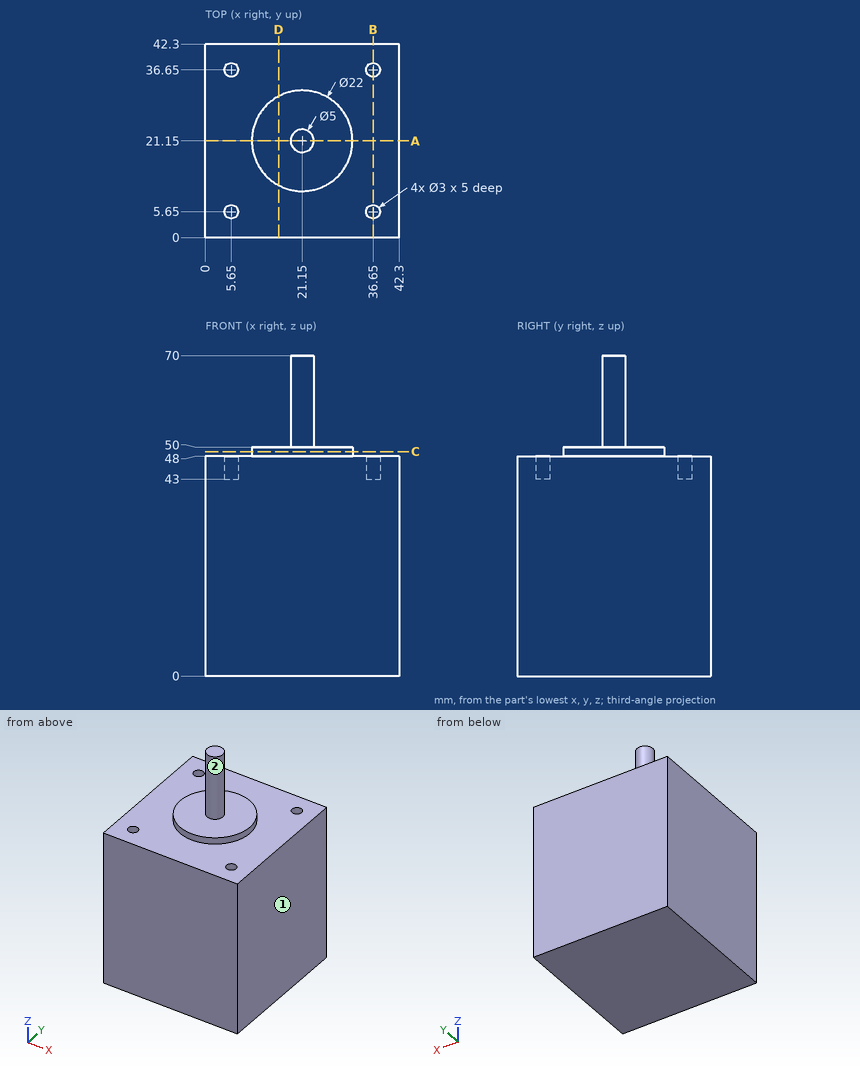
Answer from the drawing. Dimensions are ordinates in mm from the lowest x, y and z of the part. A direction names the side the tool comes from. Round coordinates to 2 decimals unless told otherwise and drop trailing zeros. Write each loop counter-clockwise with the first axis right and the second up, starting at its lowest first coordinate (ties: lowest second). Pieces come first, ordered by that corner, then holes. Notation, with made-up numbers: (27, 69) -> (46, 69) arc R23 ccw to (46, 98) -> close; hole circle Ø11 at (4.25, 88). An arc over 180 degrees is marked (long way). Answer in a Markdown table with one row per item. Add a question column.
1) Find section D-D, the plane x = 16. Determine the outline of the cut face in (y, z).
2) Find section A-A, the plane y = 21.15. Determine the outline of the cut face in (x, z), and give its area (3 significant figures).
3) Find section B-B, the plane x = 36.65. Determine the outline of the cut face in (y, z).
4) Given P1, Ø10, axis at y = 11, z = 52.5, coming from the +X side; P2, Ø8, axis at x = 22, y = 13, coming from the +Z side; P3, Ø4, axis at y = 26, z = 59.5, coming from the -X side; P4, Ø2.5, axis at x = 36.65, y = 36.65, coming from the +Z side, each flat-ended and moving along its own axis, determine where each tip first touches the part or whether it passes through.
5) Which of the six approach directions +Z, -Z, +X, -X, +Y, -Y give full straight-line access (tool end or side, diameter ignored) to the marked faces 1 and 2?
6) Consider line 1 (Y direction, x = 5.65, z = 44.15); line 2 (Z direction, x = 2, y = 26); line 3 (X direction, y = 36, z = 44). Determine where each line is inside the solid, lowest interval first.
7) Find section C-C, the plane z = 49. Determine the outline of the cut face in (x, y).
Findings below:
| question | item | result |
|---|---|---|
| 1 | outline | (0, 0) -> (42.3, 0) -> (42.3, 48) -> (30.87, 48) -> (30.87, 50) -> (11.43, 50) -> (11.43, 48) -> (0, 48) -> close |
| 2 | outline | (0, 0) -> (42.3, 0) -> (42.3, 48) -> (32.15, 48) -> (32.15, 50) -> (23.65, 50) -> (23.65, 70) -> (18.65, 70) -> (18.65, 50) -> (10.15, 50) -> (10.15, 48) -> (0, 48) -> close |
| 2 | area | 2,170 mm² |
| 3 | outline | (0, 0) -> (42.3, 0) -> (42.3, 48) -> (38.15, 48) -> (38.15, 43) -> (35.15, 43) -> (35.15, 48) -> (7.15, 48) -> (7.15, 43) -> (4.15, 43) -> (4.15, 48) -> (0, 48) -> close |
| 4 | P1 | x = 42.3 |
| 4 | P2 | z = 50 |
| 4 | P3 | through |
| 4 | P4 | z = 43 |
| 5 | face 1 | +Z, -Z, +X, +Y, -Y |
| 5 | face 2 | +Z |
| 6 | line 1 | 0 to 4.15, 7.15 to 35.15, 38.15 to 42.3 |
| 6 | line 2 | 0 to 48 |
| 6 | line 3 | 0 to 4.3, 7 to 35.3, 38 to 42.3 |
| 7 | outline | circle Ø22 at (21.15, 21.15) |
